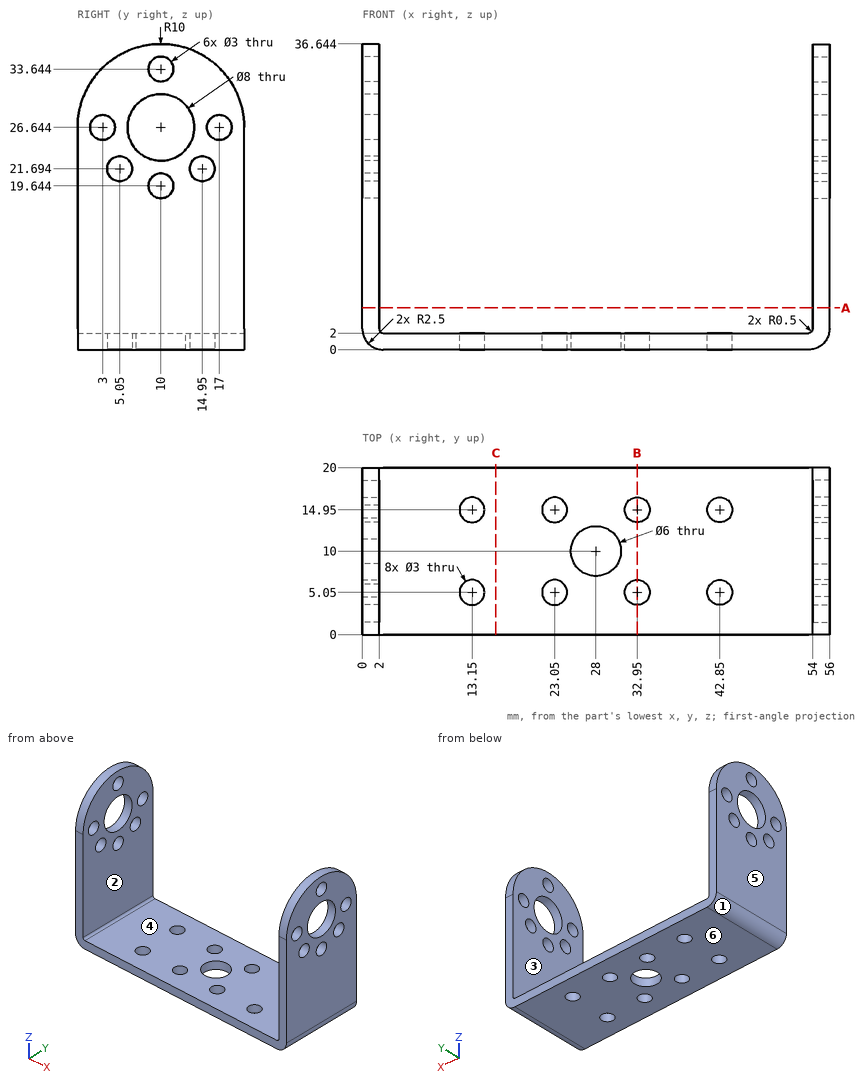
Study the drawing (mm; zero at the part's minimum x, y, z) and answer. A direction names the side the tool comes from. Coordinates: 2 decimals unless noted, no trailing zeros. Loops run counter-clockwise (first coordinate to the right, second up) from the corner with the lowest first, then second, coordinate; pieces in that order, holes last. Notation, with made-up numbers: M -7.5,2.5 L 12.5,2.5 A31 cw 12.5,41.5 Z; hole C -19,59 d3. An arc over 180 degrees is marked long. Answer as a JSON object with one key per item and string values. Group by question number.
Item 1: Section B-B (x = 32.95) is taken. Write down the section's boundary in (y, z), and give its area (3 significant figures).
Item 2: Which of the six approach directions +Z, -Z, +X, -X, +Y, -Y give full straight-line access (tool end or side, diameter ignored) to the marked faces 1 and 2?
Item 3: Determine the mould class of the marked faces 3, 4, 5 and 6 for opening direction X: +X half, -X half, draft (parallel to the pull), parting line (faces both ways), or undercut.
Item 4: Consider L1, parallel to Y at x = 42.85, z = 1.2; L2, parallel to X at y = 12, z = 19; L3, parallel to Z at x = 21, y = 16.5. Determine where each line is inside the solid, lowest interval first.
Item 5: Section A-A (z = 5) is taken. Write down the section's boundary in (x, y), and give its area (3 significant figures).
Item 6: This flat-tipped pin is pushed along its axis until it touches: P1, Ø5, axis at x = 42.85, y = 14.95, coming from the +Z side. Where does it stop, or does it pass through?
Item 7: Section C-C (x = 16) is taken. Write down the section's boundary in (y, z), and give its area (3 significant figures).
Solved:
{
 "1": {"outline": "M 0,0 L 3.55,0 L 3.55,2 L 0,2 Z; M 6.55,0 L 13.45,0 L 13.45,2 L 6.55,2 Z; M 16.45,0 L 20,0 L 20,2 L 16.45,2 Z", "area": "28.0 mm2"},
 "2": {"face 1": "-Z, -X, +Y, -Y", "face 2": "+Z, +Y, -Y"},
 "3": {"face 3": "undercut", "face 4": "undercut", "face 5": "-X half", "face 6": "draft"},
 "4": {"L1": "y = 0 to 3.55, 6.55 to 13.45, 16.45 to 20", "L2": "x = 0 to 2, 54 to 56", "L3": "z = 0 to 2"},
 "5": {"outline": "M 0,0 L 2,0 L 2,20 L 0,20 Z; M 54,0 L 56,0 L 56,20 L 54,20 Z", "area": "80.0 mm2"},
 "6": {"P1": "stops at z = 2"},
 "7": {"outline": "M 0,0 L 20,0 L 20,2 L 0,2 Z", "area": "40.0 mm2"}
}
